Part print with two shaded views. Sizes in mm from the minimum x, y, z corner. A direction names the side the tool comes from. Coordinates: 2 decimals unless noted, no trailing zeros. Loops run counter-clockwise (first coordinate to the right, second up) from the corner with the lowest first, then second, coordinate; pieces in that order, holes last.
(1) Two-plate mould, pull along X, no slides. Class the marked faces 1, 2 and 3: pulls with the +X half, pulls with the -X half, needs draft (parallel to the pull), parting line crosses it, or undercut.
(2) Slice it at D-D (y = 2.4). Give the number of separate pieces and of enclosed holes in the cut face, and give its area (3 significant figures).
(3) Wall check: L1, parallel to Z at x = 28, y = 4.1; L2, parallel to Z at x = 20, y = 3.95 (3 decimals); L3, parallel to X at y = 3.2, z = 35 (3 decimals). Give the ranges that are in metal, low to high.
(4) Tool access for the marked faces 4 and 5: list every direction of +Z, -Z, +X, -X, +Y, -Y with a clear straight run to the whole face (end or side of a thin tool).
(5) Slice it at C-C (x = 28). Give the cut face in (y, z).
(6) Slice it at A-A (x = 20). Give the cut face in (y, z) (3 decimals), and give its area (3 significant figures).
(7) Slice it at B-B (z = 35). Give the cut face in (x, y) (3 decimals), and give its area (3 significant figures).
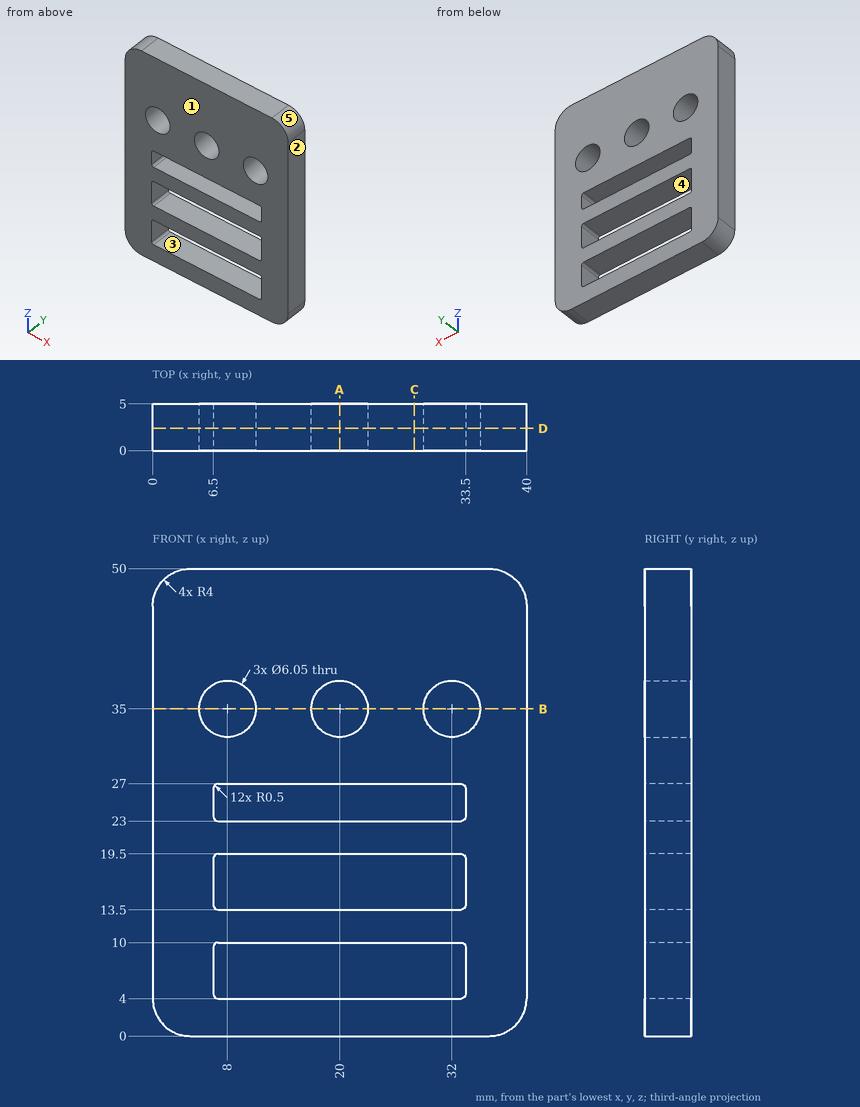
Response values:
1. face 1: needs draft
1. face 2: pulls with the +X half
1. face 3: undercut
2. separate pieces: 1
2. enclosed holes: 6
2. area: 1,470 mm2
3. L1: z = 0 to 4, 10 to 13.5, 19.5 to 23, 27 to 50
3. L2: z = 0 to 4, 10 to 13.5, 19.5 to 23, 27 to 31.975, 38.025 to 50
3. L3: x = 0 to 4.975, 11.025 to 16.975, 23.025 to 28.975, 35.025 to 40
4. face 4: +Y, -Y
4. face 5: +Z, +X, +Y, -Y
5. outline: (0, 0) - (5, 0) - (5, 4) - (0, 4) - close; (0, 10) - (5, 10) - (5, 13.5) - (0, 13.5) - close; (0, 19.5) - (5, 19.5) - (5, 23) - (0, 23) - close; (0, 27) - (5, 27) - (5, 50) - (0, 50) - close
6. outline: (0, 0) - (5, 0) - (5, 4) - (0, 4) - close; (0, 10) - (5, 10) - (5, 13.5) - (0, 13.5) - close; (0, 19.5) - (5, 19.5) - (5, 23) - (0, 23) - close; (0, 27) - (5, 27) - (5, 31.975) - (0, 31.975) - close; (0, 38.025) - (5, 38.025) - (5, 50) - (0, 50) - close
6. area: 140 mm2
7. outline: (0, 0) - (4.975, 0) - (4.975, 5) - (0, 5) - close; (11.025, 0) - (16.975, 0) - (16.975, 5) - (11.025, 5) - close; (23.025, 0) - (28.975, 0) - (28.975, 5) - (23.025, 5) - close; (35.025, 0) - (40, 0) - (40, 5) - (35.025, 5) - close
7. area: 109 mm2
